Model file for the job. Use its own axes, mm. A direction names the side the tool comes from. Round coordinates to 2 decimals unless told otherwise and drop trailing zeros. Loops run counter-clockwise (first coordinate to the right, second up) from the corner with the lowest first, then second, coordinate; pieces in that order, holes last. Notation, with made-up numbers: (-20.75, 80.5) - (29.25, 80.5) arc R17 cw to (29.25, 87.5) - close; hole circle Ø11 at (45.25, 31). An arc over 180 degrees is marked (long way). Answer as a JSON object with one key per item and string values.
from build123d import *

# Parameters (mm, degrees)
F0_R     = 0.635
F4_DEPTH = 5.08
F6_DEPTH = 19.05


with BuildPart() as f2:
    # F2: sweep along a path in F1
    with BuildLine(Plane.YZ) as f2_path:
        Line((0, 0), (0, 12.7))
        Line((0, 12.7), (12.7, 12.7))
        Line((12.7, 12.7), (12.7, 25.4))
    # F0 (on Top) → F2 (sweep)
    with BuildSketch(Plane.XY):
        Circle(F0_R)
    sweep(path=f2_path.line, transition=Transition.RIGHT)

    # F3 (on face) → F4 (join)
    with BuildSketch(Plane.XY.offset(25.4)):
        with BuildLine():
            ThreePointArc((-0.9525, 14.3497783942), (-1.3470384182, 14.0470384182), (-1.6497783942, 13.6525))
            Line((-1.6497783942, 13.6525), (-0.5499261314, 13.0175))
            ThreePointArc((-0.5499261314, 13.0175), (-0.4490128061, 13.1490128061), (-0.3175, 13.2499261314))
            Line((-0.3175, 13.2499261314), (-0.9525, 14.3497783942))
        make_face()
        with BuildLine():
            ThreePointArc((-0.3175, 13.2499261314), (-0.1643500936, 13.3133628997), (0, 13.335))
            Line((0, 13.335), (0, 14.605))
            ThreePointArc((0, 14.605), (-0.4930502809, 14.5400886991), (-0.9525, 14.3497783942))
            Line((-0.9525, 14.3497783942), (-0.3175, 13.2499261314))
        make_face()
        with BuildLine():
            Line((0, 14.605), (-1.5875, 15.449630657))
            Line((-1.5875, 15.449630657), (-0.9525, 14.3497783942))
            ThreePointArc((-0.9525, 14.3497783942), (-0.4930502809, 14.5400886991), (0, 14.605))
        make_face()
        with BuildLine():
            Line((-0.9525, 14.3497783942), (-1.5875, 15.449630657))
            Line((-1.5875, 15.449630657), (-1.6497783942, 13.6525))
            ThreePointArc((-1.6497783942, 13.6525), (-1.3470384182, 14.0470384182), (-0.9525, 14.3497783942))
        make_face()
        with BuildLine():
            Line((-0.3175, 13.2499261314), (0, 12.7))
            Line((0, 12.7), (0, 13.335))
            ThreePointArc((0, 13.335), (-0.1643500936, 13.3133628997), (-0.3175, 13.2499261314))
        make_face()
        with BuildLine():
            Line((-0.5499261314, 12.3825), (0, 12.7))
            Line((0, 12.7), (-0.635, 12.7))
            ThreePointArc((-0.635, 12.7), (-0.6133628997, 12.5356499064), (-0.5499261314, 12.3825))
        make_face()
        with BuildLine():
            Line((-0.635, 12.7), (0, 12.7))
            Line((0, 12.7), (-0.5499261314, 13.0175))
            ThreePointArc((-0.5499261314, 13.0175), (-0.6133628997, 12.8643500936), (-0.635, 12.7))
        make_face()
        with BuildLine():
            Line((-0.5499261314, 13.0175), (0, 12.7))
            Line((0, 12.7), (-0.3175, 13.2499261314))
            ThreePointArc((-0.3175, 13.2499261314), (-0.4490128061, 13.1490128061), (-0.5499261314, 13.0175))
        make_face()
        with BuildLine():
            Line((-0.3175, 12.1500738686), (0, 12.7))
            Line((0, 12.7), (-0.5499261314, 12.3825))
            ThreePointArc((-0.5499261314, 12.3825), (-0.4490128061, 12.2509871939), (-0.3175, 12.1500738686))
        make_face()
        with BuildLine():
            Line((0, 12.7), (0, 12.065))
            ThreePointArc((0, 12.065), (0.1643500936, 12.0866371003), (0.3175, 12.1500738686))
            Line((0.3175, 12.1500738686), (0, 12.7))
        make_face()
        with BuildLine():
            Line((0.5499261314, 12.3825), (0, 12.7))
            Line((0, 12.7), (0.3175, 12.1500738686))
            ThreePointArc((0.3175, 12.1500738686), (0.4490128061, 12.2509871939), (0.5499261314, 12.3825))
        make_face()
        with BuildLine():
            Line((0.635, 12.7), (0, 12.7))
            Line((0, 12.7), (0.5499261314, 12.3825))
            ThreePointArc((0.5499261314, 12.3825), (0.6133628997, 12.5356499064), (0.635, 12.7))
        make_face()
        with BuildLine():
            Line((0.5499261314, 13.0175), (0, 12.7))
            Line((0, 12.7), (0.635, 12.7))
            ThreePointArc((0.635, 12.7), (0.6133628997, 12.8643500936), (0.5499261314, 13.0175))
        make_face()
        with BuildLine():
            Line((0.3175, 13.2499261314), (0, 12.7))
            Line((0, 12.7), (0.5499261314, 13.0175))
            ThreePointArc((0.5499261314, 13.0175), (0.4490128061, 13.1490128061), (0.3175, 13.2499261314))
        make_face()
        with BuildLine():
            Line((0, 13.335), (0, 12.7))
            Line((0, 12.7), (0.3175, 13.2499261314))
            ThreePointArc((0.3175, 13.2499261314), (0.1643500936, 13.3133628997), (0, 13.335))
        make_face()
        with BuildLine():
            ThreePointArc((-0.3175, 12.1500738686), (-0.1643500936, 12.0866371003), (0, 12.065))
            Line((0, 12.065), (0, 12.7))
            Line((0, 12.7), (-0.3175, 12.1500738686))
        make_face()
        with BuildLine():
            ThreePointArc((0, 13.335), (0.1643500936, 13.3133628997), (0.3175, 13.2499261314))
            Line((0.3175, 13.2499261314), (0.9525, 14.3497783942))
            ThreePointArc((0.9525, 14.3497783942), (0.4930502809, 14.5400886991), (0, 14.605))
            Line((0, 14.605), (0, 13.335))
        make_face()
        with BuildLine():
            Line((0.5499261314, 13.0175), (1.6497783942, 13.6525))
            ThreePointArc((1.6497783942, 13.6525), (1.3470384182, 14.0470384182), (0.9525, 14.3497783942))
            Line((0.9525, 14.3497783942), (0.3175, 13.2499261314))
            ThreePointArc((0.3175, 13.2499261314), (0.4490128061, 13.1490128061), (0.5499261314, 13.0175))
        make_face()
        with BuildLine():
            Line((0.9525, 14.3497783942), (1.5875, 15.449630657))
            Line((1.5875, 15.449630657), (0, 14.605))
            ThreePointArc((0, 14.605), (0.4930502809, 14.5400886991), (0.9525, 14.3497783942))
        make_face()
        with BuildLine():
            Line((1.6497783942, 13.6525), (1.5875, 15.449630657))
            Line((1.5875, 15.449630657), (0.9525, 14.3497783942))
            ThreePointArc((0.9525, 14.3497783942), (1.3470384182, 14.0470384182), (1.6497783942, 13.6525))
        make_face()
        with BuildLine():
            Line((0.635, 12.7), (1.905, 12.7))
            ThreePointArc((1.905, 12.7), (1.8400886991, 13.1930502809), (1.6497783942, 13.6525))
            Line((1.6497783942, 13.6525), (0.5499261314, 13.0175))
            ThreePointArc((0.5499261314, 13.0175), (0.6133628997, 12.8643500936), (0.635, 12.7))
        make_face()
        with BuildLine():
            Line((0.5499261314, 12.3825), (1.6497783942, 11.7475))
            ThreePointArc((1.6497783942, 11.7475), (1.8400886991, 12.2069497191), (1.905, 12.7))
            Line((1.905, 12.7), (0.635, 12.7))
            ThreePointArc((0.635, 12.7), (0.6133628997, 12.5356499064), (0.5499261314, 12.3825))
        make_face()
        with BuildLine():
            Line((0.3175, 12.1500738686), (0.9525, 11.0502216058))
            ThreePointArc((0.9525, 11.0502216058), (1.3470384182, 11.3529615818), (1.6497783942, 11.7475))
            Line((1.6497783942, 11.7475), (0.5499261314, 12.3825))
            ThreePointArc((0.5499261314, 12.3825), (0.4490128061, 12.2509871939), (0.3175, 12.1500738686))
        make_face()
        with BuildLine():
            Line((0, 12.065), (0, 10.795))
            ThreePointArc((0, 10.795), (0.4930502809, 10.8599113009), (0.9525, 11.0502216058))
            Line((0.9525, 11.0502216058), (0.3175, 12.1500738686))
            ThreePointArc((0.3175, 12.1500738686), (0.1643500936, 12.0866371003), (0, 12.065))
        make_face()
        with BuildLine():
            ThreePointArc((-0.9525, 11.0502216058), (-0.4930502809, 10.8599113009), (0, 10.795))
            Line((0, 10.795), (0, 12.065))
            ThreePointArc((0, 12.065), (-0.1643500936, 12.0866371003), (-0.3175, 12.1500738686))
            Line((-0.3175, 12.1500738686), (-0.9525, 11.0502216058))
        make_face()
        with BuildLine():
            ThreePointArc((-1.6497783942, 11.7475), (-1.3470384182, 11.3529615818), (-0.9525, 11.0502216058))
            Line((-0.9525, 11.0502216058), (-0.3175, 12.1500738686))
            ThreePointArc((-0.3175, 12.1500738686), (-0.4490128061, 12.2509871939), (-0.5499261314, 12.3825))
            Line((-0.5499261314, 12.3825), (-1.6497783942, 11.7475))
        make_face()
        with BuildLine():
            ThreePointArc((-1.905, 12.7), (-1.8400886991, 12.2069497191), (-1.6497783942, 11.7475))
            Line((-1.6497783942, 11.7475), (-0.5499261314, 12.3825))
            ThreePointArc((-0.5499261314, 12.3825), (-0.6133628997, 12.5356499064), (-0.635, 12.7))
            Line((-0.635, 12.7), (-1.905, 12.7))
        make_face()
        with BuildLine():
            ThreePointArc((-1.6497783942, 13.6525), (-1.8400886991, 13.1930502809), (-1.905, 12.7))
            Line((-1.905, 12.7), (-0.635, 12.7))
            ThreePointArc((-0.635, 12.7), (-0.6133628997, 12.8643500936), (-0.5499261314, 13.0175))
            Line((-0.5499261314, 13.0175), (-1.6497783942, 13.6525))
        make_face()
        with BuildLine():
            Line((-1.6497783942, 13.6525), (-3.175, 12.7))
            Line((-3.175, 12.7), (-1.905, 12.7))
            ThreePointArc((-1.905, 12.7), (-1.8400886991, 13.1930502809), (-1.6497783942, 13.6525))
        make_face()
        with BuildLine():
            Line((-1.905, 12.7), (-3.175, 12.7))
            Line((-3.175, 12.7), (-1.6497783942, 11.7475))
            ThreePointArc((-1.6497783942, 11.7475), (-1.8400886991, 12.2069497191), (-1.905, 12.7))
        make_face()
        with BuildLine():
            Line((-1.6497783942, 11.7475), (-1.5875, 9.950369343))
            Line((-1.5875, 9.950369343), (-0.9525, 11.0502216058))
            ThreePointArc((-0.9525, 11.0502216058), (-1.3470384182, 11.3529615818), (-1.6497783942, 11.7475))
        make_face()
        with BuildLine():
            Line((-1.5875, 9.950369343), (0, 10.795))
            ThreePointArc((0, 10.795), (-0.4930502809, 10.8599113009), (-0.9525, 11.0502216058))
            Line((-0.9525, 11.0502216058), (-1.5875, 9.950369343))
        make_face()
        with BuildLine():
            ThreePointArc((0.9525, 11.0502216058), (0.4930502809, 10.8599113009), (0, 10.795))
            Line((0, 10.795), (1.5875, 9.950369343))
            Line((1.5875, 9.950369343), (0.9525, 11.0502216058))
        make_face()
        with BuildLine():
            Line((0.9525, 11.0502216058), (1.5875, 9.950369343))
            Line((1.5875, 9.950369343), (1.6497783942, 11.7475))
            ThreePointArc((1.6497783942, 11.7475), (1.3470384182, 11.3529615818), (0.9525, 11.0502216058))
        make_face()
        with BuildLine():
            Line((1.6497783942, 11.7475), (3.175, 12.7))
            Line((3.175, 12.7), (1.905, 12.7))
            ThreePointArc((1.905, 12.7), (1.8400886991, 12.2069497191), (1.6497783942, 11.7475))
        make_face()
        with BuildLine():
            Line((1.905, 12.7), (3.175, 12.7))
            Line((3.175, 12.7), (1.6497783942, 13.6525))
            ThreePointArc((1.6497783942, 13.6525), (1.8400886991, 13.1930502809), (1.905, 12.7))
        make_face()
    extrude(amount=F4_DEPTH)

    # F5 (on face) → F6 (join)
    with BuildSketch(Plane.XY.offset(30.48)):
        with BuildLine():
            ThreePointArc((0.635, 12.7), (-0.4490128061, 13.1490128061), (0, 12.065))
            Line((0, 12.065), (0, 12.7))
            Line((0, 12.7), (0.635, 12.7))
        make_face()
        with BuildLine():
            Line((0, 12.7), (0, 12.065))
            ThreePointArc((0, 12.065), (0.4490128061, 12.2509871939), (0.635, 12.7))
            Line((0.635, 12.7), (0, 12.7))
        make_face()
    extrude(amount=F6_DEPTH)


solid = f2.part
1) Probe probe 1 along Y at (x, z) = (0, 21.5) (3 decimals); probe 2 along Z at (x, y) = (-0.5, 13.5); probe 3 along X at (y, z) = (10, 12.5). List the from-to ranges inside material, lowest first.
Values follow:
{"probe 1": "12.065 to 13.335", "probe 2": "25.4 to 30.48", "probe 3": "-0.6 to 0.6"}
2) Tool access for faces 5 (the cylindrical face through (-0.08, 13.33, 18.83)), 6 (the flat face through (0.8, 15.03, 27.9)), 7 (the flat face through (0.78, 10.38, 27.9)), 8 (the cylindrical face through (-0.14, -0.62, 6.76)): list every direction of +Z, -Z, +X, -X, +Y, -Y with a clear straight run to the whole face (end or side of a thin tool).
Values follow:
{"face 5": "none", "face 6": "+Z, -Z, +Y", "face 7": "+Z, -Y", "face 8": "-Z"}
3) Drop flat-ended pins along their axis: P1, Ø1.5, axis at x = 0, y = 11.5, coming from the -Z side (3 decimals); P2, Ø1.5, axis at x = -1.5, z = 40.5, coming from the +Y side; P3, Ø8, axis at y = 9.5, z = 26.5, coming from the -X side (3 decimals). Give the stop position or say it passes through.
Values follow:
{"P1": "z = 12.065", "P2": "through", "P3": "x = -3.175"}
4) Slice it at D-D on z = 12.7. List the corners of the cut face in (x, y) (3 decimals).
Values follow:
{"outline": "(-0.635, 0) arc R0.635 ccw to (0.635, 0) - (0.635, 12.7) arc R0.635 ccw to (-0.635, 12.7) - close"}
5) Slice it at C-C on y = 0. List the corners of the cut face in (x, z) (3 decimals).
Values follow:
{"outline": "(-0.635, 0) - (0.635, 0) - (0.635, 12.7) arc R0.635 ccw to (-0.635, 12.7) - close"}
6) Two-plate mould, pull along X, no slides. Class faces 1 (the flat face through (-0.78, 15.02, 27.9)), 2 (the flat face through (-2.402, 13.183, 27.904)), 3 (the flat face through (2.42, 13.17, 27.9)), 4 (the flat face through (1, 13, 25.4)): pulls with the +X half, pulls with the -X half, needs draft (parallel to the pull), parting line crosses it, or undercut.
Values follow:
{"face 1": "undercut", "face 2": "pulls with the -X half", "face 3": "pulls with the +X half", "face 4": "needs draft"}
7) Slice it at A-A on z = 22.5. List the corners of the cut face in (x, y) (3 decimals).
Values follow:
{"outline": "circle Ø1.27 at (0, 12.7)"}
